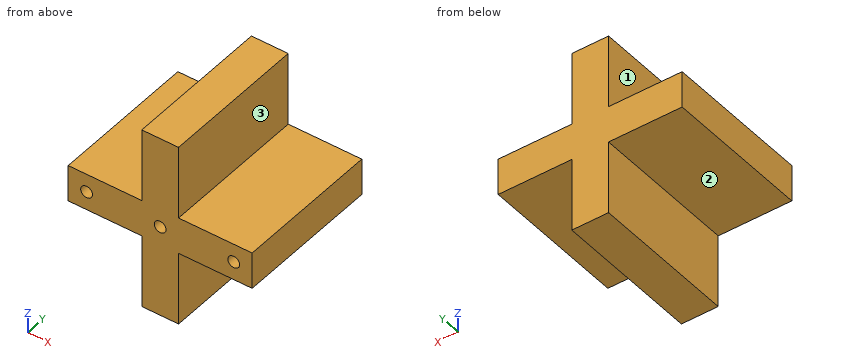
from build123d import *

# Parameters (mm, degrees)
CRUZ_DEPTH                 = 100
CROQUIS_AGUJEROS_MONTAJE_R = 4
AGUJERO_INSERTO_M6_DEPTH   = 14


with BuildPart() as part:
    # Croquis_cruz → Cruz (new body)
    with BuildSketch(Plane(origin=(0, 0, 0), x_dir=(1, 0, 0), z_dir=(0, 1, 0))):
        Polygon((-62.5, -12.5), (-12.5, -12.5), (-12.5, -62.5), (12.5, -62.5), (12.5, -12.5), (62.5, -12.5), (62.5, 12.5), (12.5, 12.5), (12.5, 62.5), (-12.5, 62.5), (-12.5, 12.5), (-62.5, 12.5), align=None)
    extrude(amount=CRUZ_DEPTH)

    # Croquis_agujeros_montaje → Agujero_inserto_M6 (cut)
    with BuildSketch(Plane(origin=(0, 0, 0), x_dir=(1, 0, 0), z_dir=(0, 1, 0))):
        with Locations(Location((-50, 0, 0), (0, 0, 270))):
            Circle(CROQUIS_AGUJEROS_MONTAJE_R)
        with Locations(Location((0, 0, 0), (0, 0, 270))):
            Circle(CROQUIS_AGUJEROS_MONTAJE_R)
        with Locations(Location((50, 0, 0), (0, 0, 270))):
            Circle(CROQUIS_AGUJEROS_MONTAJE_R)
    extrude(amount=AGUJERO_INSERTO_M6_DEPTH, mode=Mode.SUBTRACT)


solid = part.part
For this review, take the finished solid that the model builds, in its own axes (mm). Face numbers are marked on the shaded views. A direction names the side the tool comes from. Give positions to 0.01 mm unless a question says otherwise; leave off trailing zeros. Loops run counter-clockwise (first coordinate to the right, second up) from the corner with the lowest first, then second, coordinate; pieces in that order, holes last. Notation, with made-up numbers: M 89,-7.75 L 144,-7.75 A37 cw 144,28.25 Z; hole C 17,49.25 d5. An arc over 180 degrees is marked long. Answer as a JSON object with one key per item and string values. Group by question number.
Q1. Add section C-C on y = 35. Give the boundary of the cut face in (x, z).
Q2. Insertion check: P1, Ø10, axis at x = -33, z = -6, coming from the -Y side; P2, Ø5, axis at x = -50, z = 0, coming from the -Y side; P3, Ø15, axis at y = 37, z = -42, coming from the +X side; P4, Ø2, axis at x = -21, y = 51.5, coming from the -Z side. Each pin has a flat end and moves straight along its axis. Give the tip position at first contact, or say it passes through.
Q3. For probe 1 along X at (y, z) = (3.5, 0); probe 2 along X at (y, z) = (71.5, -54), list the stretches that pass through material, from the lowest coordinate up. Write a range as [from, to].
Q4. Tool access review of the marked faces 1, 2 and 3: name each direction out of +Z, -Z, +X, -X, +Y, -Y from which nothing blocks a thin tool from reaching the whole face with its end or side.
Q5. Add section A-A on x = 50. Give the boundary of the cut face in (y, z).
Q6. Add section B-B on z = 0. Give the boundary of the cut face in (x, y), and give its area (3 significant figures).
Q7. Add section D-D on z = 16.5. Give the boundary of the cut face in (x, y).
Checked values:
{
 "1": {"outline": "M -62.5,-12.5 L -12.5,-12.5 L -12.5,-62.5 L 12.5,-62.5 L 12.5,-12.5 L 62.5,-12.5 L 62.5,12.5 L 12.5,12.5 L 12.5,62.5 L -12.5,62.5 L -12.5,12.5 L -62.5,12.5 Z"},
 "2": {"P1": "y = 0", "P2": "y = 14", "P3": "x = 12.5", "P4": "z = -12.5"},
 "3": {"probe 1": "[-62.5, -54], [-46, -4], [4, 46], [54, 62.5]", "probe 2": "[-12.5, 12.5]"},
 "4": {"face 1": "+Z, -X, +Y, -Y", "face 2": "-Z, -X, +Y, -Y", "face 3": "+Z, +X, +Y, -Y"},
 "5": {"outline": "M 0,-12.5 L 100,-12.5 L 100,12.5 L 0,12.5 L 0,4 L 14,4 L 14,-4 L 0,-4 Z"},
 "6": {"outline": "M -62.5,0 L -54,0 L -54,14 L -46,14 L -46,0 L -4,0 L -4,14 L 4,14 L 4,0 L 46,0 L 46,14 L 54,14 L 54,0 L 62.5,0 L 62.5,100 L -62.5,100 Z", "area": "12,200 mm²"},
 "7": {"outline": "M -12.5,0 L 12.5,0 L 12.5,100 L -12.5,100 Z"}
}
